Work out the finished part from the listing and answer in its coordinate system (mm). A direction names the side the tool comes from. Round coordinates to 2 decimals unless told otherwise and drop trailing zeros. Write each loop counter-clockwise with the first axis right and the second up, starting at its lowest first coordinate (ties: lowest second). Pieces come first, ordered by that corner, then holes.
1. A tool of negligible diameter and unlimited length cuts with its end or side. For faces 1 (the face through (-1.521, -13.183, -13.23)), 2 (the face through (-2, -13, 14.5)), 3 (the face through (0, -14.5, 0)), 4 (the face through (-2, -12.5, 1)), 5 (the face through (21, -7.5, 21)), from which of +Z, -Z, +X, -X, +Y, -Y can it reach the whole face along a straight path? Write none if from no direction.
2. Find section B-B (y = -4.25). Write down the section's boundary in (x, z), and give its area (3 significant figures).
3. Find section A-A (z = 0). Write down the section's boundary in (x, y).
4. Flat-ended cylindrical pins translate along their axes: pin 1 Ø3 at (x, z) = (7.5, 11) entering from -Y; pin 2 Ø1.4 at (y, z) = (1, 0) entering from -X; pin 3 Ø3 at (y, z) = (4, -5.5) entering from +X. Find the tip coordinate at first contact, or state that the pin passes through.
5. Determine the mould class of faces 6 (the face through (1.98, 1.39, -0.89)), 7 (the face through (2.7, -0.1, -14.5)), 8 (the face through (7, 9.395, 0)) for opening direction Y: pulls with the +Y half, pulls with the -Y half, needs draft (parallel to the pull), parting line crosses it, or undercut.
6. Find section C-C (z = 6.5). Write down the section's boundary in (x, y).
7. Straight lines are drawn through the part: probe 1 along Y at (x, z) = (1.55, 0); probe 2 along Y at (x, z) = (7.5, -3); probe 3 along X at (y, z) = (-9.5, 11.5). For each, find the intervals that lie inside material, in ascending order.
8. Find section D-D (y = -1). Write down the section's boundary in (x, z).
```python
from build123d import *

# Parameters (mm, degrees)
EXTRUDE_1_DEPTH        = 5
EXTRUDE_1_DEPTH_BACK   = 3
SKETCH_2_W             = 29
SKETCH_2_H             = 29
SKETCH_3_W             = 25
SKETCH_3_H             = 25
CUT_EXTRUDE_1_DEPTH    = 3
SKETCH_5_R             = 1
CUT_EXTRUDE_3_DEPTH    = 3
CUT_EXTRUDE_4_DEPTH    = 23.011360703
HOLE_WIZARD_M4_1_D     = 3.3
HOLE_WIZARD_M4_1_DEPTH = 10.1
HOLE_WIZARD_M4_1_TIP   = 0.991420021
SKETCH_4_W             = 8
SKETCH_4_H             = 29
EXTRUDE_2_DEPTH        = 13.4052
SKETCH_7_W             = 29
SKETCH_7_H             = 5
EXTRUDE_3_DEPTH        = 5
SKETCH_10_W            = 29
SKETCH_10_H            = 13.4052
CUT_EXTRUDE_5_DEPTH    = 35.028667136
EXTRUDE_4_DEPTH        = 28
SKETCH_13_W            = 22.441758485
SKETCH_13_H            = 29
CUT_EXTRUDE_7_DEPTH    = 20.8948
SKETCH_14_W            = 27
SKETCH_14_H            = 6.1052
CUT_EXTRUDE_8_DEPTH    = 10
EXTRUDE_5_DEPTH        = 10
SKETCH_16_W            = 12.441758485
SKETCH_16_H            = 20.8948
CUT_EXTRUDE_9_DEPTH    = 5
CUT_EXTRUDE_10_DEPTH   = 5
SKETCH_18_W            = 7.441758485
SKETCH_18_H            = 20.8948
CUT_EXTRUDE_11_DEPTH   = 1.9068532
SKETCH_19_W            = 18
SKETCH_19_H            = 8
CUT_EXTRUDE_12_DEPTH   = 7
SKETCH_20_W            = 3.0931468
SKETCH_20_H            = 11
EXTRUDE_6_DEPTH        = 20
SKETCH_21_W            = 3.0931468
SKETCH_21_H            = 2.8948
CUT_EXTRUDE_13_DEPTH   = 7.441758485
SKETCH_22_W            = 29
SKETCH_22_H            = 7
CUT_EXTRUDE_14_DEPTH   = 7.558241515
EXTRUDE_7_DEPTH        = 3
SKETCH_24_W            = 3
SKETCH_24_H            = 11
CUT_EXTRUDE_15_DEPTH   = 50.942466899
CUT_EXTRUDE_16_DEPTH   = 3.8082415
SKETCH_26_W            = 11.249999985
SKETCH_26_H            = 6.1052
CUT_EXTRUDE_17_DEPTH   = 6.0931468
SKETCH_27_W            = 6.0931468
SKETCH_27_H            = 6.1052
CUT_EXTRUDE_18_DEPTH   = 43.86096708
CUT_EXTRUDE_19_DEPTH   = 3.1052
SKETCH_30_W            = 3.750000015
SKETCH_30_H            = 32.721043552
CUT_EXTRUDE_20_DEPTH   = 7.8948
CUT_EXTRUDE_21_DEPTH   = 4.9068532
SKETCH_32_W            = 31.249999985
SKETCH_32_H            = 6.0931468
CUT_EXTRUDE_22_DEPTH   = 3.5
SKETCH_33_W            = 11
SKETCH_33_H            = 13.8948
EXTRUDE_8_DEPTH        = 3
SKETCH_34_W            = 11
SKETCH_34_H            = 6.3948
CUT_EXTRUDE_25_DEPTH   = 49.005208051
EXTRUDE_9_DEPTH        = 0.3948
SKETCH_36_W            = 38
SKETCH_36_H            = 7.8948
CUT_EXTRUDE_26_DEPTH   = 2.5931468
CUT_EXTRUDE_27_DEPTH   = 3.5
SKETCH_38_W            = 1.185809648
SKETCH_38_H            = 4.3948
CUT_EXTRUDE_28_DEPTH   = 3.750000015
EXTRUDE_11_DEPTH       = 3
EXTRUDE_12_REACH       = 51.952


with BuildPart() as part:
    # 草图2 → 凸台-拉伸1 (new, two sides: drawn at the far end of the back side and taken through both)
    with BuildSketch(Plane(origin=(0, 0, 0), x_dir=(0, 0, -1), z_dir=(1, 0, 0)).offset(-EXTRUDE_1_DEPTH_BACK)):
        Rectangle(SKETCH_2_W, SKETCH_2_H)
    extrude(amount=EXTRUDE_1_DEPTH + EXTRUDE_1_DEPTH_BACK)

    # 草图3 → 切除-拉伸1 (cut)
    with BuildSketch(Plane.ZY.offset(3)):
        Rectangle(SKETCH_3_W, SKETCH_3_H)
    extrude(amount=-CUT_EXTRUDE_1_DEPTH, mode=Mode.SUBTRACT)

    # 草图5 → 切除-拉伸3 (cut)
    with BuildSketch(Plane.ZY.offset(3)):
        with Locations((-12.5, -12.5)):
            Circle(SKETCH_5_R)
    extrude(amount=-CUT_EXTRUDE_3_DEPTH, mode=Mode.SUBTRACT)

    # 草图6 → 切除-拉伸4 (cut, through all)
    with BuildSketch(Plane.ZY.offset(3)):
        Polygon((12.5, 12.5), (12.5, -12.5), (14.5, -12.5), (14.5, 14.5), (-12.5, 14.5), (-14.5, 14.5), (-14.5, 12.5), (-12.5, 12.5), align=None)
    extrude(amount=-CUT_EXTRUDE_4_DEPTH, mode=Mode.SUBTRACT)

    # M4 螺纹孔1
    with Locations(Plane.ZY):
        with Locations((0, 0)):
            Hole(HOLE_WIZARD_M4_1_D / 2, depth=HOLE_WIZARD_M4_1_DEPTH)
            with Locations((0, 0, -(HOLE_WIZARD_M4_1_DEPTH + HOLE_WIZARD_M4_1_TIP / 2))):  # 118° drill point
                Cone(0, HOLE_WIZARD_M4_1_D / 2, HOLE_WIZARD_M4_1_TIP, mode=Mode.SUBTRACT)

    # 草图4 → 凸台-拉伸2 (add)
    with BuildSketch(Plane.XZ.offset(14.5)):
        with Locations((1, 0)):
            Rectangle(SKETCH_4_W, SKETCH_4_H)
    extrude(amount=EXTRUDE_2_DEPTH)

    # 草图7 → 凸台-拉伸3 (add)
    with BuildSketch(Plane(origin=(5, 0, 0), x_dir=(0, 0, -1), z_dir=(1, 0, 0))):
        with Locations((0, -25.4052)):
            Rectangle(SKETCH_7_W, SKETCH_7_H)
    extrude(amount=EXTRUDE_3_DEPTH)

    # 草图10 → 切除-拉伸5 (cut, through all)
    with BuildSketch(Plane.ZY.offset(3)):
        with Locations((0, -21.2026)):
            Rectangle(SKETCH_10_W, SKETCH_10_H)
    extrude(amount=-CUT_EXTRUDE_5_DEPTH, mode=Mode.SUBTRACT)

    # 草图12 → 凸台-拉伸4 (add)
    with BuildSketch(Plane(origin=(5, 0, 0), x_dir=(0, 0, -1), z_dir=(1, 0, 0))):
        Polygon((-14.5, -14.5), (14.5, -14.5), (14.5, 12.5), (-12.5, 12.5), (-12.5, -12.5), (-14.5, -12.5), align=None)
    extrude(amount=EXTRUDE_4_DEPTH)

    # 草图13 → 切除-拉伸7 (cut)
    with BuildSketch(Plane.XZ.offset(14.5)):
        with Locations((21.779120757, 0)):
            Rectangle(SKETCH_13_W, SKETCH_13_H)
    extrude(amount=-CUT_EXTRUDE_7_DEPTH, mode=Mode.SUBTRACT)

    # 草图14 → 切除-拉伸8 (cut)
    with BuildSketch(Plane(origin=(33, 0, 0), x_dir=(0, 0, -1), z_dir=(1, 0, 0))):
        with Locations((1, 9.4474)):
            Rectangle(SKETCH_14_W, SKETCH_14_H)
    extrude(amount=-CUT_EXTRUDE_8_DEPTH, mode=Mode.SUBTRACT)

    # 草图15 → 凸台-拉伸5 (add)
    with BuildSketch(Plane.XY.offset(12.5)):
        Polygon((23, 6.3948), (23, 12.5), (0, 12.5), (0, -14.5), (23, -14.5), align=None)
    extrude(amount=EXTRUDE_5_DEPTH)

    # 草图16 → 切除-拉伸9 (cut)
    with BuildSketch(Plane(origin=(0, 0, 12.5), x_dir=(-1, 0, 0), z_dir=(0, 0, -1))):
        with Locations((-16.779120757, -4.0526)):
            Rectangle(SKETCH_16_W, SKETCH_16_H)
    extrude(amount=-CUT_EXTRUDE_9_DEPTH, mode=Mode.SUBTRACT)

    # 草图17 → 切除-拉伸10 (cut)
    with BuildSketch(Plane(origin=(23, 0, 0), x_dir=(0, 0, -1), z_dir=(1, 0, 0))):
        Polygon((-17.5, -14.5), (-17.5, 6.3948), (14.5, 6.3948), (14.5, 12.5), (-22.5, 12.5), (-22.5, -14.5), align=None)
    extrude(amount=-CUT_EXTRUDE_10_DEPTH, mode=Mode.SUBTRACT)

    # 草图18 → 切除-拉伸11 (cut)
    with BuildSketch(Plane(origin=(0, 0, 17.5), x_dir=(-1, 0, 0), z_dir=(0, 0, -1))):
        with Locations((-14.279120757, -4.0526)):
            Rectangle(SKETCH_18_W, SKETCH_18_H)
    extrude(amount=-CUT_EXTRUDE_11_DEPTH, mode=Mode.SUBTRACT)

    # 草图19 → 切除-拉伸12 (cut)
    with BuildSketch(Plane.XZ.offset(14.5)):
        with Locations((9, 18.5)):
            Rectangle(SKETCH_19_W, SKETCH_19_H)
    extrude(amount=-CUT_EXTRUDE_12_DEPTH, mode=Mode.SUBTRACT)

    # 草图20 → 凸台-拉伸6 (add)
    with BuildSketch(Plane(origin=(18, 0, 0), x_dir=(0, 0, -1), z_dir=(1, 0, 0))):
        with Locations((-20.9534266, -2)):
            Rectangle(SKETCH_20_W, SKETCH_20_H)
    extrude(amount=EXTRUDE_6_DEPTH)

    # 草图21 → 切除-拉伸13 (cut)
    with BuildSketch(Plane(origin=(18, 0, 0), x_dir=(0, 0, -1), z_dir=(1, 0, 0))):
        with Locations((-20.9534266, 4.9474)):
            Rectangle(SKETCH_21_W, SKETCH_21_H)
    extrude(amount=-CUT_EXTRUDE_13_DEPTH, mode=Mode.SUBTRACT)

    # 草图22 → 切除-拉伸14 (cut)
    with BuildSketch(Plane(origin=(10.558241515, 0, 0), x_dir=(0, 0, -1), z_dir=(1, 0, 0))):
        with Locations((0, -11)):
            Rectangle(SKETCH_22_W, SKETCH_22_H)
    extrude(amount=-CUT_EXTRUDE_14_DEPTH, mode=Mode.SUBTRACT)

    # 草图23 → 凸台-拉伸7 (add)
    with BuildSketch(Plane.XY.offset(22.5)):
        Polygon((10.558241515, 6.3948), (18, 6.3948), (18, 12.5), (0, 12.5), (0, -7.5), (38, -7.5), (38, 3.5), (10.558241515, 3.5), align=None)
    extrude(amount=EXTRUDE_7_DEPTH)

    # 草图24 → 切除-拉伸15 (cut, through all)
    with BuildSketch(Plane.XZ.offset(7.5)):
        with Locations((1.5, 20)):
            Rectangle(SKETCH_24_W, SKETCH_24_H)
    extrude(amount=-CUT_EXTRUDE_15_DEPTH, mode=Mode.SUBTRACT)

    # 草图25 → 切除-拉伸16 (cut)
    with BuildSketch(Plane(origin=(10.558241515, 0, 0), x_dir=(0, 0, -1), z_dir=(1, 0, 0))):
        Polygon((-19.4068532, -7.5), (14.5, -7.5), (14.5, 6.3948), (-25.5, 6.3948), (-25.5, 3.5), (-19.4068532, 3.5), align=None)
    extrude(amount=-CUT_EXTRUDE_16_DEPTH, mode=Mode.SUBTRACT)

    # 草图26 → 切除-拉伸17 (cut)
    with BuildSketch(Plane.XY.offset(25.5)):
        with Locations((12.375000008, 9.4474)):
            Rectangle(SKETCH_26_W, SKETCH_26_H)
    extrude(amount=-CUT_EXTRUDE_17_DEPTH, mode=Mode.SUBTRACT)

    # 草图27 → 切除-拉伸18 (cut, through all)
    with BuildSketch(Plane(origin=(6.750000015, 0, 0), x_dir=(0, 0, -1), z_dir=(1, 0, 0))):
        with Locations((-22.4534266, 9.4474)):
            Rectangle(SKETCH_27_W, SKETCH_27_H)
    extrude(amount=-CUT_EXTRUDE_18_DEPTH, mode=Mode.SUBTRACT)

    # 草图28 → 切除-拉伸19 (cut)
    with BuildSketch(Plane(origin=(0, 12.5, 0), x_dir=(1, 0, 0), z_dir=(0, 1, 0))):
        Polygon((3, -14.5), (3, -19.4068532), (18, -19.4068532), (18, 14.5), (-3, 14.5), (-3, 12.5), (0, 12.5), (0, -14.5), align=None)
    extrude(amount=-CUT_EXTRUDE_19_DEPTH, mode=Mode.SUBTRACT)

    # 草图30 → 切除-拉伸20 (cut)
    with BuildSketch(Plane.XZ.offset(7.5)):
        with Locations((4.875000008, 1.860521776)):
            Rectangle(SKETCH_30_W, SKETCH_30_H)
    extrude(amount=-CUT_EXTRUDE_20_DEPTH, mode=Mode.SUBTRACT)

    # 草图31 → 切除-拉伸21 (cut)
    with BuildSketch(Plane.XY.offset(19.4068532)):
        Polygon((18, 6.3948), (18, 9.3948), (3, 9.3948), (3, 6.3948), (6.750000015, 6.3948), align=None)
    extrude(amount=-CUT_EXTRUDE_21_DEPTH, mode=Mode.SUBTRACT)

    # 草图32 → 切除-拉伸22 (cut)
    with BuildSketch(Plane(origin=(0, 3.5, 0), x_dir=(1, 0, 0), z_dir=(0, 1, 0))):
        with Locations((22.375000007, -22.4534266)):
            Rectangle(SKETCH_32_W, SKETCH_32_H)
    extrude(amount=-CUT_EXTRUDE_22_DEPTH, mode=Mode.SUBTRACT)

    # 草图33 → 凸台-拉伸8 (add)
    with BuildSketch(Plane.ZY.offset(-3)):
        with Locations((20, -0.5526)):
            Rectangle(SKETCH_33_W, SKETCH_33_H)
    extrude(amount=EXTRUDE_8_DEPTH)

    # 草图34 → 切除-拉伸25 (cut, through all)
    with BuildSketch(Plane(origin=(0, 0, 0), x_dir=(0, 0, -1), z_dir=(1, 0, 0))):
        with Locations((-20, 3.1974)):
            Rectangle(SKETCH_34_W, SKETCH_34_H)
    extrude(amount=CUT_EXTRUDE_25_DEPTH, mode=Mode.SUBTRACT)

    # 草图35 → 凸台-拉伸9 (add)
    with BuildSketch(Plane(origin=(0, 0, 0), x_dir=(1, 0, 0), z_dir=(0, 1, 0))):
        Polygon((38, -25.5), (38, -19.4068532), (6.750000015, -19.4068532), (6.750000015, -18.221043552), (3, -18.221043552), (3, -14.5), (0, -14.5), (0, -25.5), align=None)
    extrude(amount=EXTRUDE_9_DEPTH)

    # 草图36 → 切除-拉伸26 (cut)
    with BuildSketch(Plane.XY.offset(25.5)):
        with Locations((19, -3.5526)):
            Rectangle(SKETCH_36_W, SKETCH_36_H)
    extrude(amount=-CUT_EXTRUDE_26_DEPTH, mode=Mode.SUBTRACT)

    # 草图37 → 切除-拉伸27 (cut)
    with BuildSketch(Plane(origin=(0, 0.3948, 0), x_dir=(1, 0, 0), z_dir=(0, 1, 0))):
        Polygon((3, -14.5), (0, -14.5), (0, -22.9068532), (38, -22.9068532), (38, -19.4068532), (6.750000015, -19.4068532), (6.750000015, -18.221043552), (3, -18.221043552), align=None)
    extrude(amount=-CUT_EXTRUDE_27_DEPTH, mode=Mode.SUBTRACT)

    # 草图38 → 切除-拉伸28 (cut)
    with BuildSketch(Plane(origin=(6.750000015, 0, 0), x_dir=(0, 0, -1), z_dir=(1, 0, 0))):
        with Locations((-18.813948376, -5.3026)):
            Rectangle(SKETCH_38_W, SKETCH_38_H)
    extrude(amount=-CUT_EXTRUDE_28_DEPTH, mode=Mode.SUBTRACT)

    # 草图39 → 凸台-拉伸11 (add)
    with BuildSketch(Plane(origin=(3, 0, 0), x_dir=(0, 0, -1), z_dir=(1, 0, 0))):
        Polygon((-14.5, 9.3948), (-14.5, -14.5), (-22.9068532, -7.5), (-22.9068532, -3.1052), align=None)
    extrude(amount=-EXTRUDE_11_DEPTH)

    # 凸台-拉伸12: up to this face of the body (flat: up to its plane)
    extrude_12_end = Plane(part.part.faces().sort_by_distance((1.5, 3.1448, 18.7034266))[0])
    # 草图40 → 凸台-拉伸12 (add, up to the picked face)
    with BuildSketch(Plane.XY.offset(14.5), mode=Mode.PRIVATE) as extrude_12_sk1:
        Polygon((3, 9.3948), (3, 0.3948), (6.750000015, 0.3948), (6.750000015, 6.3948), (18, 6.3948), (18, 9.3948), align=None)
    extrude_12_tool1 = split(extrude(extrude_12_sk1.sketch, amount=EXTRUDE_12_REACH, mode=Mode.PRIVATE), bisect_by=extrude_12_end, keep=Keep.BOTH, mode=Mode.PRIVATE)
    add(extrude_12_tool1.solids().sort_by(Axis((3.174929, 4.8948, 14.5), (0, 0, 1)))[0])


solid = part.part
```
Worked answers:
1. face 1: -X
1. face 2: +Z, -X, +Y, -Y
1. face 3: +Z, -Z, +X, -X, -Y
1. face 4: +Z, -X, +Y
1. face 5: +Z, -Z, +X, -Y
2. outline: (-3, -14.5) - (3, -14.5) - (3, 19.41) - (38, 19.41) - (38, 22.91) - (0, 22.91) - (0, -12.5) - (-3, -12.5) - close
2. area: 241 mm2
3. outline: (-3, -14.5) - (3, -14.5) - (3, -1.65) - (0, -1.65) - (0, -12.5) - (-3, -12.5) - close; (0, 1.65) - (5, 1.65) - (5, 0.39) - (6.75, 0.39) - (6.75, 6.39) - (18, 6.39) - (18, 9.39) - (0, 9.39) - close
4. pin 1: stops at y = 0.39
4. pin 2: stops at x = 0
4. pin 3: stops at x = 6.75
5. face 6: undercut
5. face 7: needs draft
5. face 8: pulls with the +Y half
6. outline: (-3, -14.5) - (3, -14.5) - (3, 0.39) - (6.75, 0.39) - (6.75, 6.39) - (18, 6.39) - (18, 9.39) - (0, 9.39) - (0, -12.5) - (-3, -12.5) - close
7. probe 1: y = -14.5 to -1.65, 1.65 to 9.39
7. probe 2: y = 6.39 to 9.39
7. probe 3: x = 0 to 3
8. outline: (-3, -14.5) - (3, -14.5) - (3, -1.31) - (0, -1.31) - (0, -12.5) - (-3, -12.5) - close; (0, 1.31) - (3, 1.31) - (3, 21.49) - (0, 21.49) - close
